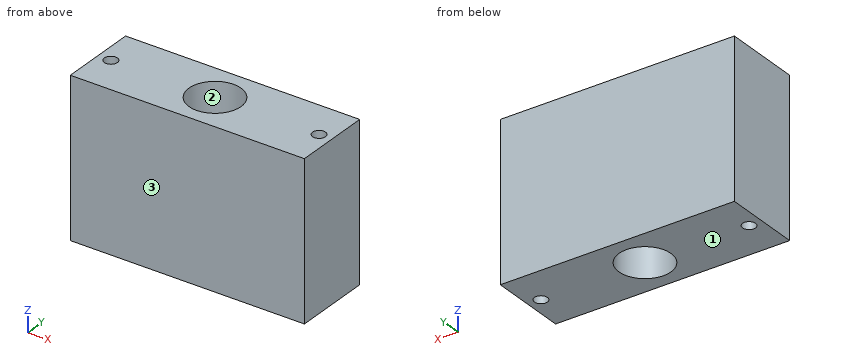
```python
from build123d import *

# Parameters (mm, degrees)
F0_W     = 114.3
F0_H     = 38.1
F1_DEPTH = 76.2
F2_R     = 12.7
F3_DEPTH = 85.598
F4_R     = 3.175
F5_DEPTH = 90.678
F6_R     = 3.175
F7_DEPTH = 90.678


with BuildPart() as f1:
    # F0 (on Top) → F1 (new body)
    with BuildSketch(Plane.XY):
        with Locations((29.87668, 19.05)):
            Rectangle(F0_W, F0_H)
    extrude(amount=F1_DEPTH)

    # F2 (on Top) → F3 (cut)
    with BuildSketch(Plane.XY):
        with Locations((29.87668, 19.05)):
            Circle(F2_R)
    extrude(amount=F3_DEPTH, mode=Mode.SUBTRACT)

    # F4 (on Top) → F5 (cut)
    with BuildSketch(Plane.XY):
        with Locations((-20.92332, 19.05)):
            Circle(F4_R)
    extrude(amount=F5_DEPTH, mode=Mode.SUBTRACT)

    # F6 (on Top) → F7 (cut)
    with BuildSketch(Plane.XY):
        with Locations((80.67668, 19.05)):
            Circle(F6_R)
    extrude(amount=F7_DEPTH, mode=Mode.SUBTRACT)


solid = f1.part
```
Build history of the part. All positions in model axes, mm. Face numbers are marked on the shaded views. Round coordinates to 2 decimals unless told otherwise and drop trailing zeros. Write each loop counter-clockwise with the first axis right and the second up, starting at its lowest first coordinate (ties: lowest second). Pieces come first, ordered by that corner, then holes. Notation, with made-up numbers: (65.25, 48) - (72.25, 48) arc R21 cw to (72.25, 82) - close; hole circle Ø10 at (8, -28.75). An arc over 180 degrees is marked (long way). Write each question's results on one line, items separated by ' | '. Start each with the question number.
Item 1: Drop a flat-ended pin along its axis: P1, Ø5, axis at x = -20.92, y = 19.05, coming from the -Z side. Give the stop position or say it passes through.
Item 2: Saw through at B-B (x = 79.5). Write the cut outline in (y, z).
Item 3: Saw through at C-C (z = 8.5). Write the cut outline in (x, y) (3 decimals).
Item 4: Mould opens along Y. For the marked faces 1, 2 and 3 say: pulls with the +Y half, pulls with the -Y half, needs draft (parallel to the pull), parting line crosses it, or undercut.
Item 5: Saw through at A-A (y = 19.05). Write the cut outline in (x, z), and give its area (3 significant figures).
Item 6: Saw through at D-D (y = 27). Write the cut outline in (x, z), and give its area (3 significant figures).
Item 7: Wall check: L1, parallel to X at y = 19.05, z = 21.5; L2, parallel to X at y = 17, z = 60.5; L3, parallel to X at y = 29, z = 49. Give the ranges that are in metal, low to high. Write a range as [from, to].
Results are:
1) P1: passes through
2) outline: (0, 0) - (16.1, 0) - (16.1, 76.2) - (0, 76.2) - close; (22, 0) - (38.1, 0) - (38.1, 76.2) - (22, 76.2) - close
3) outline: (-27.273, 0) - (87.027, 0) - (87.027, 38.1) - (-27.273, 38.1) - close; hole circle Ø6.35 at (-20.923, 19.05); hole circle Ø25.4 at (29.877, 19.05); hole circle Ø6.35 at (80.677, 19.05)
4) face 1: needs draft | face 2: undercut | face 3: pulls with the -Y half
5) outline: (-27.27, 0) - (-24.1, 0) - (-24.1, 76.2) - (-27.27, 76.2) - close; (-17.75, 0) - (17.18, 0) - (17.18, 76.2) - (-17.75, 76.2) - close; (42.58, 0) - (77.5, 0) - (77.5, 76.2) - (42.58, 76.2) - close; (83.85, 0) - (87.03, 0) - (87.03, 76.2) - (83.85, 76.2) - close | area: 5,810 mm²
6) outline: (-27.27, 0) - (19.97, 0) - (19.97, 76.2) - (-27.27, 76.2) - close; (39.78, 0) - (87.03, 0) - (87.03, 76.2) - (39.78, 76.2) - close | area: 7,200 mm²
7) L1: x = [-27.27, -24.1], [-17.75, 17.18], [42.58, 77.5], [83.85, 87.03] | L2: x = [-27.27, -23.35], [-18.5, 17.34], [42.41, 78.25], [83.1, 87.03] | L3: x = [-27.27, 21.98], [37.77, 87.03]
